Work out the finished part from the listing and answer in its coordinate system (mm). Face numbers are marked on the shaded views. Round coordinates to 2 decimals unless told otherwise and drop trailing zeros. Order: outer loops, then holes, each group sorted by start corner. A loop starts at its lowest first (then second) coordinate and runs counter-clockwise, first axis right, second up. Notation, with made-up numbers: (26, -12) - (33, -12) arc R22 ccw to (33, 3) - close; hole circle Ø11 at (-25, -35.75). An arc over 180 degrees is marked (long way). Use one line per item in the form item = value. Start each with the question number.
Q1. The part is cut by section A-A on x = 0. Determine the outline of the cut face in (y, z).
Q2. Given P1, Ø6, axis at x = -3.5, z = 3.5, coming from the +Y side; P2, Ø1.5, axis at x = -34.5, z = -12, coming from the -Y side; P3, Ø12, axis at y = -10.5, z = -28.5, coming from the -X side, each flat-ended and moving along its own axis, determine where each tip first touches the part or whether it passes through.
Q3. Find the intervals of material crossed by line 1 (Y direction, x = 0, z = 3.9); line 2 (Z direction, x = -36, y = -61); line 3 (Y direction, x = -28, z = 23), in increasing order. Write a range as [from, to].
Q4. The part is cut by section B-B on y = 0. Determine the outline of the cut face in (x, z).
Q5. For a pull along Z with two mould halves and no side action, classify the marked faces 1, 2, 3 and 4 as +Z half, -Z half, draft (parallel to the pull), parting line (faces both ways), or undercut.
Q6. The part is cut by section D-D on x = -38. Determine the outline of the cut face in (y, z), plus the area to 3 significant figures.
Q7. The part is cut by section C-C on y = -57. Determine the outline of the cut face in (x, z), plus the area to 3 significant figures.
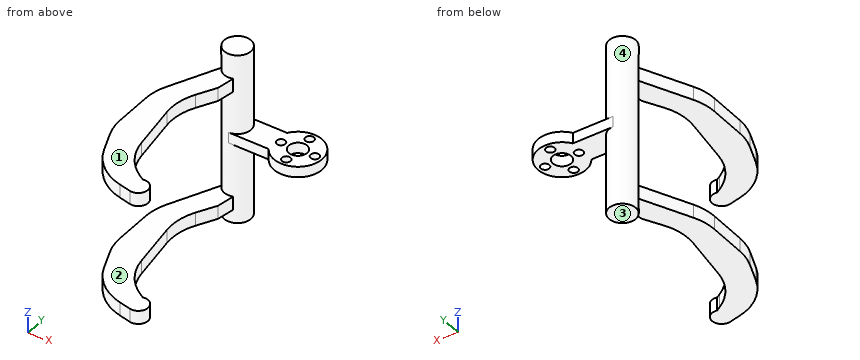
from build123d import *

# Parameters (mm, degrees)
SKETCH2_R                = 11.43
BOSS_EXTRUDE1_DEPTH      = 5.08
SKETCH4_R                = 4.318
SKETCH4_R_2              = 2.032
CUT_EXTRUDE1_DEPTH       = 5.08
BOSS_EXTRUDE2_DEPTH      = 5.08
CIRPATTERN1_COUNT        = 4
BOSS_EXTRUDE3_DEPTH      = 38.1
BOSS_EXTRUDE3_DEPTH_BACK = 43.18
SKETCH9_R                = 6.35
BOSS_EXTRUDE4_DEPTH      = 6.35
FILLET1_R                = 25.4
FILLET1_OF_MIRROR1_R     = 25.4


with BuildPart() as part:
    # Sketch2 → Boss-Extrude1 (new body)
    with BuildSketch(Plane.XY):
        Circle(SKETCH2_R)
    extrude(amount=BOSS_EXTRUDE1_DEPTH)

    # Sketch4 → Cut-Extrude1 (cut)
    with BuildSketch(Plane(origin=(0, 0, 0), x_dir=(-1, 0, 0), z_dir=(0, 0, -1))):
        Circle(SKETCH4_R)
        with Locations((0, -8.001)):
            Circle(SKETCH4_R_2)
    cut_extrude1 = extrude(amount=-CUT_EXTRUDE1_DEPTH, mode=Mode.SUBTRACT)

    # Sketch7 → Boss-Extrude2 (add)
    with BuildSketch(Plane(origin=(0, 0, 0), x_dir=(-1, 0, 0), z_dir=(0, 0, -1))):
        with BuildLine():
            Line((9.503809762, 6.35), (28.553809762, 6.35))
            ThreePointArc((28.553809762, 6.35), (34.903809762, 0), (28.553809762, -6.35))
            Line((28.553809762, -6.35), (9.503809762, -6.35))
            Line((9.503809762, -6.35), (9.503809762, 6.35))
        make_face()
    extrude(amount=-BOSS_EXTRUDE2_DEPTH)

    # CirPattern1: Cut-Extrude1 ×4 about axis
    cirpattern1_axis = Axis((0, 0, 0), (0, 0, 1))
    for i in range(1, CIRPATTERN1_COUNT):
        add(cut_extrude1.rotate(cirpattern1_axis, i * 360 / CIRPATTERN1_COUNT), mode=Mode.SUBTRACT)

    # Sketch9 → Boss-Extrude3 (add, two sides: drawn at the far end of the back side and taken through both)
    with BuildSketch(Plane.XY.offset(5.08).offset(-BOSS_EXTRUDE3_DEPTH_BACK)):
        with Locations((-28.553809762, 0)):
            Circle(SKETCH9_R)
    extrude(amount=BOSS_EXTRUDE3_DEPTH + BOSS_EXTRUDE3_DEPTH_BACK)

    # Sketch12 → Boss-Extrude4 (add)
    with BuildSketch(Plane.XY.offset(-31.75)):
        with BuildLine():
            Line((-25.378809762, 0), (-33.047894508, 0))
            Line((-33.047894508, 0), (-47.267412368, -30.245447294))
            Line((-47.267412368, -30.245447294), (-47.267412368, -58.33420365))
            Line((-47.267412368, -58.33420365), (-36.57534741, -84.867934272))
            Line((-36.57534741, -84.867934272), (-18.073665796, -88.9))
            ThreePointArc((-18.073665796, -88.9), (-12.52460446, -84.430000607), (-18.073665796, -79.960001215))
            Line((-18.073665796, -79.960001215), (-30.345802798, -72.608060715))
            Line((-30.345802798, -72.608060715), (-36.57534741, -30.245447294))
            Line((-36.57534741, -30.245447294), (-27.94, -14.249719927))
            Line((-27.94, -14.249719927), (-25.378809762, 0))
        make_face()
    boss_extrude4 = extrude(amount=BOSS_EXTRUDE4_DEPTH)

    # Fillet1
    fillet1_edges = [part.edges().sort_by_distance(p)[0] for p in [
        (-36.57534741, -84.867934272, -28.575),
        (-30.345802798, -72.608060715, -28.575),
        (-36.57534741, -30.245447294, -28.575),
        (-47.267412368, -30.245447294, -28.575),
        (-47.267412368, -58.33420365, -28.575),
    ]]
    fillet(fillet1_edges, radius=FILLET1_R)

    # Mirror1: Boss-Extrude4 across plane
    add(boss_extrude4.mirror(Plane.XY))

    # Fillet1 of Mirror1
    fillet1_of_mirror1_edges = [part.edges().sort_by_distance(p)[0] for p in [
        (-36.57534741, -84.867934272, 28.575),
        (-30.345802798, -72.608060715, 28.575),
        (-36.57534741, -30.245447294, 28.575),
        (-47.267412368, -30.245447294, 28.575),
        (-47.267412368, -58.33420365, 28.575),
    ]]
    fillet(fillet1_of_mirror1_edges, radius=FILLET1_OF_MIRROR1_R)


solid = part.part
Found:
q1.outline = (-11.43, 0) - (-10.03, 0) - (-10.03, 5.08) - (-11.43, 5.08) - close; (-5.97, 0) - (-4.32, 0) - (-4.32, 5.08) - (-5.97, 5.08) - close; (4.32, 0) - (5.97, 0) - (5.97, 5.08) - (4.32, 5.08) - close; (10.03, 0) - (11.43, 0) - (11.43, 5.08) - (10.03, 5.08) - close
q2.P1 = 11.42
q2.P2 = -3.65
q2.P3 = -40.81
q3.line_1 = [-11.43, -10.03], [-5.97, -4.32], [4.32, 5.97], [10.03, 11.43]
q3.line_2 = [-31.75, -25.4], [25.4, 31.75]
q3.line_3 = [-6.33, 6.33]
q4.outline = (-34.9, -38.1) - (-22.2, -38.1) - (-22.2, 0) - (-10.03, 0) - (-10.03, 5.08) - (-22.2, 5.08) - (-22.2, 43.18) - (-34.9, 43.18) - close; (-5.97, 0) - (-4.32, 0) - (-4.32, 5.08) - (-5.97, 5.08) - close; (4.32, 0) - (5.97, 0) - (5.97, 5.08) - (4.32, 5.08) - close; (10.03, 0) - (11.43, 0) - (11.43, 5.08) - (10.03, 5.08) - close
q5.face_1 = +Z half
q5.face_2 = undercut
q5.face_3 = -Z half
q5.face_4 = undercut
q6.outline = (-78.62, -31.75) - (-10.53, -31.75) - (-10.53, -25.4) - (-78.62, -25.4) - close; (-78.62, 25.4) - (-10.53, 25.4) - (-10.53, 31.75) - (-78.62, 31.75) - close
q6.area = 865 mm²
q7.outline = (-47.01, -31.75) - (-32.64, -31.75) - (-32.64, -25.4) - (-47.01, -25.4) - close; (-47.01, 25.4) - (-32.64, 25.4) - (-32.64, 31.75) - (-47.01, 31.75) - close
q7.area = 183 mm²
